The model under review builds one solid part; all positions refer to its coordinate system, in mm. A direction names the side the tool comes from. Coordinates: 2 decimals unless noted, no trailing zeros. Order: outer loops, then holes, each group sorted by start corner. A loop starts at its lowest first (then second) coordinate and runs counter-clockwise, first axis right, second up. Notation, with made-up numbers: M -36.75,82 L 22.25,82 A19 cw 22.25,117 Z; hole C -30,24 d1. An arc over 180 degrees is marked long. One line per item, written item: value.
```python
from build123d import *

# Parameters (mm, degrees)
EXTRUDE_1_DEPTH = 20


with BuildPart() as part:
    # 草图2 → 凸台-拉伸1 (new body)
    with BuildSketch(Plane.XY):
        with BuildLine():
            Line((-1.042752475, -10.085861632), (3.857247525, -10.085861632))
            ThreePointArc((3.857247525, -10.085861632), (4.757247525, -10.985861632), (3.857247525, -11.885861632))
            Line((3.857247525, -11.885861632), (1.076161722, -11.885861632))
            ThreePointArc((1.076161722, -11.885861632), (0.722608332, -12.032308241), (0.576161722, -12.385861632))
            Line((0.576161722, -12.385861632), (0.576161722, -12.790788968))
            ThreePointArc((0.576161722, -12.790788968), (0.614221956, -12.982130685), (0.722608332, -13.144342359))
            Line((0.722608332, -13.144342359), (2.885447948, -15.307181975))
            ThreePointArc((2.885447948, -15.307181975), (3.858717994, -15.957500229), (5.006768291, -16.185861632))
            Line((5.006768291, -16.185861632), (8.907726758, -16.185861632))
            ThreePointArc((8.907726758, -16.185861632), (10.055777055, -15.957500229), (11.029047102, -15.307181975))
            Line((11.029047102, -15.307181975), (13.191886718, -13.144342359))
            ThreePointArc((13.191886718, -13.144342359), (13.300273094, -12.982130685), (13.338333327, -12.790788968))
            Line((13.338333327, -12.790788968), (13.338333327, -12.385861632))
            ThreePointArc((13.338333327, -12.385861632), (13.191886718, -12.032308241), (12.838333327, -11.885861632))
            Line((12.838333327, -11.885861632), (10.057247525, -11.885861632))
            ThreePointArc((10.057247525, -11.885861632), (9.157247525, -10.985861632), (10.057247525, -10.085861632))
            Line((10.057247525, -10.085861632), (14.957247525, -10.085861632))
            ThreePointArc((14.957247525, -10.085861632), (16.371461087, -10.671648069), (16.957247525, -12.085861632))
            Line((16.957247525, -12.085861632), (16.957247525, -16.985861632))
            ThreePointArc((16.957247525, -16.985861632), (16.057247525, -17.885861632), (15.157247525, -16.985861632))
            Line((15.157247525, -16.985861632), (15.157247525, -14.204775829))
            ThreePointArc((15.157247525, -14.204775829), (15.010800915, -13.851222438), (14.657247525, -13.704775829))
            Line((14.657247525, -13.704775829), (14.252320188, -13.704775829))
            ThreePointArc((14.252320188, -13.704775829), (14.060978472, -13.742836063), (13.898766797, -13.851222438))
            Line((13.898766797, -13.851222438), (11.735927181, -16.014062054))
            ThreePointArc((11.735927181, -16.014062054), (11.085608927, -16.987332101), (10.857247525, -18.135382398))
            Line((10.857247525, -18.135382398), (10.857247525, -22.036340865))
            ThreePointArc((10.857247525, -22.036340865), (11.085608927, -23.184391162), (11.735927181, -24.157661209))
            Line((11.735927181, -24.157661209), (13.898766797, -26.320500825))
            ThreePointArc((13.898766797, -26.320500825), (14.060978472, -26.4288872), (14.252320188, -26.466947434))
            Line((14.252320188, -26.466947434), (14.657247525, -26.466947434))
            ThreePointArc((14.657247525, -26.466947434), (15.010800915, -26.320500825), (15.157247525, -25.966947434))
            Line((15.157247525, -25.966947434), (15.157247525, -23.185861632))
            ThreePointArc((15.157247525, -23.185861632), (16.057247525, -22.285861632), (16.957247525, -23.185861632))
            Line((16.957247525, -23.185861632), (16.957247525, -28.085861632))
            ThreePointArc((16.957247525, -28.085861632), (16.371461087, -29.500075194), (14.957247525, -30.085861632))
            Line((14.957247525, -30.085861632), (10.057247525, -30.085861632))
            ThreePointArc((10.057247525, -30.085861632), (9.157247525, -29.185861632), (10.057247525, -28.285861632))
            Line((10.057247525, -28.285861632), (12.838333327, -28.285861632))
            ThreePointArc((12.838333327, -28.285861632), (13.191886718, -28.139415022), (13.338333327, -27.785861632))
            Line((13.338333327, -27.785861632), (13.338333327, -27.380934295))
            ThreePointArc((13.338333327, -27.380934295), (13.300273094, -27.189592579), (13.191886718, -27.027380904))
            Line((13.191886718, -27.027380904), (11.029047102, -24.864541288))
            ThreePointArc((11.029047102, -24.864541288), (10.055777055, -24.214223034), (8.907726758, -23.985861632))
            Line((8.907726758, -23.985861632), (5.006768291, -23.985861632))
            ThreePointArc((5.006768291, -23.985861632), (3.858717994, -24.214223034), (2.885447948, -24.864541288))
            Line((2.885447948, -24.864541288), (0.722608332, -27.027380904))
            ThreePointArc((0.722608332, -27.027380904), (0.614221956, -27.189592579), (0.576161722, -27.380934295))
            Line((0.576161722, -27.380934295), (0.576161722, -27.785861632))
            ThreePointArc((0.576161722, -27.785861632), (0.722608332, -28.139415022), (1.076161722, -28.285861632))
            Line((1.076161722, -28.285861632), (3.857247525, -28.285861632))
            ThreePointArc((3.857247525, -28.285861632), (4.757247525, -29.185861632), (3.857247525, -30.085861632))
            Line((3.857247525, -30.085861632), (-1.042752475, -30.085861632))
            ThreePointArc((-1.042752475, -30.085861632), (-2.456966038, -29.500075194), (-3.042752475, -28.085861632))
            Line((-3.042752475, -28.085861632), (-3.042752475, -23.185861632))
            ThreePointArc((-3.042752475, -23.185861632), (-2.142752475, -22.285861632), (-1.242752475, -23.185861632))
            Line((-1.242752475, -23.185861632), (-1.242752475, -25.966947434))
            ThreePointArc((-1.242752475, -25.966947434), (-1.096305866, -26.320500825), (-0.742752475, -26.466947434))
            Line((-0.742752475, -26.466947434), (-0.337825138, -26.466947434))
            ThreePointArc((-0.337825138, -26.466947434), (-0.146483422, -26.4288872), (0.015728252, -26.320500825))
            Line((0.015728252, -26.320500825), (2.178567868, -24.157661209))
            ThreePointArc((2.178567868, -24.157661209), (2.828886122, -23.184391162), (3.057247525, -22.036340865))
            Line((3.057247525, -22.036340865), (3.057247525, -18.135382398))
            ThreePointArc((3.057247525, -18.135382398), (2.828886122, -16.987332101), (2.178567868, -16.014062054))
            Line((2.178567868, -16.014062054), (0.015728252, -13.851222438))
            ThreePointArc((0.015728252, -13.851222438), (-0.146483422, -13.742836063), (-0.337825138, -13.704775829))
            Line((-0.337825138, -13.704775829), (-0.742752475, -13.704775829))
            ThreePointArc((-0.742752475, -13.704775829), (-1.096305866, -13.851222438), (-1.242752475, -14.204775829))
            Line((-1.242752475, -14.204775829), (-1.242752475, -16.985861632))
            ThreePointArc((-1.242752475, -16.985861632), (-2.142752475, -17.885861632), (-3.042752475, -16.985861632))
            Line((-3.042752475, -16.985861632), (-3.042752475, -12.085861632))
            ThreePointArc((-3.042752475, -12.085861632), (-2.456966038, -10.671648069), (-1.042752475, -10.085861632))
        make_face()
    extrude(amount=EXTRUDE_1_DEPTH)


solid = part.part
```
(1) For L1, parallel to X at y = -12.5, z = 17.5; L2, parallel to Y at x = -0.5, z = 6.5; L3, parallel to Y at x = 9.75, z = 10.5, list the stretches that pass through material, from the lowest coordinate up.
Geometry results:
L1: x = -3.04 to 0.58, 13.34 to 16.96
L2: y = -30.09 to -26.47, -13.7 to -10.09
L3: y = -30.03 to -28.34, -24.11 to -16.07, -11.83 to -10.14
(2) We need section A-A, the plane x = 12.25. State the section outline as (y, z) points.
Geometry results:
outline: M -30.09,0 L -28.29,0 L -28.29,20 L -30.09,20 Z; M -26.09,0 L -24.67,0 L -24.67,20 L -26.09,20 Z; M -15.5,0 L -14.09,0 L -14.09,20 L -15.5,20 Z; M -11.89,0 L -10.09,0 L -10.09,20 L -11.89,20 Z
(3) We need section C-C, the plane y = -21. State the section outline as (x, z) points, plus the area to 3 significant figures.
Geometry results:
outline: M 3.06,0 L 10.86,0 L 10.86,20 L 3.06,20 Z
area: 156 mm2
(4) Tool access review of faces 1 (the flat face through (7, -23.986, 10)), 2 (the cylindrical face through (16.39, -29.48, 9.86)), 3 (the flat face through (11, -11.886, 10)): name each direction out of +Z, -Z, +X, -X, +Y, -Y from which nothing blocks a thin tool from reaching the whole face with its end or side.
Geometry results:
face 1: +Z, -Z, -Y
face 2: +Z, -Z, +X, -Y
face 3: +Z, -Z
(5) Insertion check: pin 1 Ø4.5 at (x, z) = (7.5, 13.5) entering from +Y; pin 2 Ø4.5 at (y, z) = (-21, 10) entering from +X; pin 3 Ø1.2 at (y, z) = (-19.5, 11) entering from -X; pin 4 Ø1 at (y, z) = (-19.5, 7) entering from +X. Each pin has a flat end and moves straight along its axis. Give the tip position at first contact, or say it passes through.
Geometry results:
pin 1: stops at y = -10.14
pin 2: stops at x = 16.96
pin 3: stops at x = 3.06
pin 4: stops at x = 10.86
(6) We need section B-B, the plane y = -15. State the section outline as (x, z) points, plus the area to 3 significant figures.
Geometry results:
outline: M -3.04,0 L -1.24,0 L -1.24,20 L -3.04,20 Z; M 1.16,0 L 2.58,0 L 2.58,20 L 1.16,20 Z; M 11.34,0 L 12.75,0 L 12.75,20 L 11.34,20 Z; M 15.16,0 L 16.96,0 L 16.96,20 L 15.16,20 Z
area: 129 mm2
(7) Mouldability with a two-part tool opening along X and no side actions: class faces 4 (the cylindrical face through (2.835, -17.003, 9.86)), 5 (the cylindrical face through (3.87, -24.21, 9.86)), 6 (the flat face through (7, -20, 0)), 7 (the cylindrical face through (-2.441, -29.516, 9.86)) as +X half, -X half, draft (parallel to the pull), parting line (faces both ways), or undercut.
Geometry results:
face 4: undercut
face 5: undercut
face 6: draft
face 7: -X half
